```python
from build123d import *

# Parameters (mm, degrees)
SKETCH_1_W          = 7.8
SKETCH_1_H          = 7.8
EXTRUDE_1_DEPTH     = 9.6
SKETCH_2_R          = 2.4
EXTRUDE_2_DEPTH     = 1.7
SKETCH_3_R          = 2.5
CUT_EXTRUDE_1_DEPTH = 1.8
SKETCH_5_R          = 2.4
EXTRUDE_3_DEPTH     = 1.7


with BuildPart() as part:
    # Эскиз1 → Бобышка-Вытянуть1 (new body)
    with BuildSketch(Plane.XY):
        Rectangle(SKETCH_1_W, SKETCH_1_H)
    extrude(amount=EXTRUDE_1_DEPTH)

    # Эскиз2 → Бобышка-Вытянуть2 (add)
    with BuildSketch(Plane(origin=(0, 0, 0), x_dir=(-1, 0, 0), z_dir=(0, 0, -1))):
        Circle(SKETCH_2_R)
    extrude(amount=EXTRUDE_2_DEPTH)

    # Эскиз3 → Вырез-Вытянуть1 (cut)
    with BuildSketch(Plane.XY.offset(9.6)):
        Circle(SKETCH_3_R)
    extrude(amount=-CUT_EXTRUDE_1_DEPTH, mode=Mode.SUBTRACT)

    # Эскиз5 → Бобышка-Вытянуть3 (add)
    with BuildSketch(Plane(origin=(0, 3.9, 0), x_dir=(1, 0, 0), z_dir=(0, 1, 0))):
        with Locations(Location((0, -3.9, 0), (0, 0, 270))):
            Circle(SKETCH_5_R)
    extrude(amount=EXTRUDE_3_DEPTH)


solid = part.part
```
The model under review builds one solid part; all positions refer to its coordinate system, in mm. A direction names the side the tool comes from. Give positions to 0.01 mm unless a question says otherwise; leave off trailing zeros. Write each loop counter-clockwise with the first axis right and the second up, starting at its lowest first coordinate (ties: lowest second). Pieces come first, ordered by that corner, then holes.
(1) Tool access review of faces 4 (the flat face through (-3.9, 0, 5)), 5 (the cylindrical face through (-0.54, -2.44, 8.71)), 6 (the flat face through (-2, 2, 0)), 7 (the flat face through (0, 3.9, 7)): name each direction out of +Z, -Z, +X, -X, +Y, -Y from which nothing blocks a thin tool from reaching the whole face with its end or side.
(2) Consider section D-D, the plane y = 0. Give the boundary of the cut face in (x, z), and give its area (3 significant figures).
(3) Consider section C-C, the plane z = 3.9. Give the boundary of the cut face in (x, y), and give its area (3 significant figures).
(4) Consider section B-B, the plane y = 1. Give the boundary of the cut face in (x, z).
(5) The part is to be moulded in two halves that separate along X. For faces 1 (the cylindrical face through (0.72, 4.74, 6.19)), 2 (the flat face through (0, 0, 7.8)), 3 (the flat face through (0, 5.6, 4)), say which applies: released by +X, released by -X, zero draft, split by the parting line, or undercut.
(6) To check wall thickness, follow L1, parallel to Y at x = 0, z = 8.6; L2, parallel to Z at x = 2.25, y = 1; L3, parallel to Z at x = -1.25, y = -3. State the ranges of each line that lie inside material, in increasing order.
(7) Consider section A-A, the plane x = 0. Give the boundary of the cut face in (y, z), and give its area (3 significant figures).
Returned:
1. face 4: +Z, -Z, -X, +Y, -Y
1. face 5: +Z
1. face 6: -Z
1. face 7: +Y
2. outline: (-3.9, 0) - (-2.4, 0) - (-2.4, -1.7) - (2.4, -1.7) - (2.4, 0) - (3.9, 0) - (3.9, 9.6) - (2.5, 9.6) - (2.5, 7.8) - (-2.5, 7.8) - (-2.5, 9.6) - (-3.9, 9.6) - close
2. area: 74.0 mm2
3. outline: (-3.9, -3.9) - (3.9, -3.9) - (3.9, 3.9) - (2.4, 3.9) - (2.4, 5.6) - (-2.4, 5.6) - (-2.4, 3.9) - (-3.9, 3.9) - close
3. area: 69.0 mm2
4. outline: (-3.9, 0) - (-2.18, 0) - (-2.18, -1.7) - (2.18, -1.7) - (2.18, 0) - (3.9, 0) - (3.9, 9.6) - (2.29, 9.6) - (2.29, 7.8) - (-2.29, 7.8) - (-2.29, 9.6) - (-3.9, 9.6) - close
5. face 1: split by the parting line
5. face 2: undercut
5. face 3: zero draft
6. L1: y = -3.9 to -2.5, 2.5 to 3.9
6. L2: z = 0 to 7.8
6. L3: z = 0 to 9.6
7. outline: (-3.9, 0) - (-2.4, 0) - (-2.4, -1.7) - (2.4, -1.7) - (2.4, 0) - (3.9, 0) - (3.9, 1.5) - (5.6, 1.5) - (5.6, 6.3) - (3.9, 6.3) - (3.9, 9.6) - (2.5, 9.6) - (2.5, 7.8) - (-2.5, 7.8) - (-2.5, 9.6) - (-3.9, 9.6) - close
7. area: 82.2 mm2
